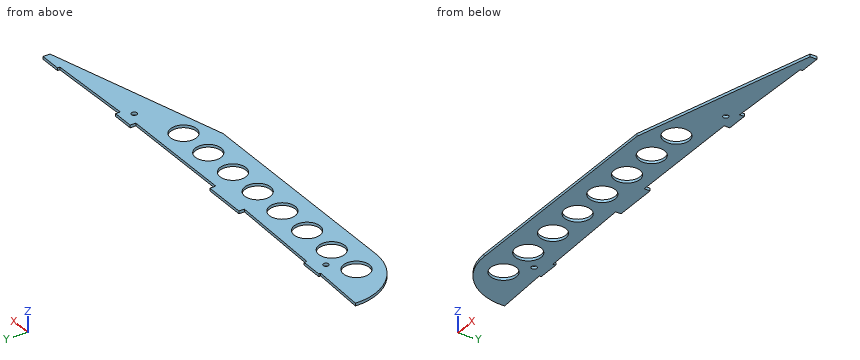
```python
from build123d import *

# Parameters (mm, degrees)
BOSS_EXTRUDE1_DEPTH      = 1.5875
BOSS_EXTRUDE1_DEPTH_BACK = 1.5875
CUT_EXTRUDE1_DEPTH       = 552.50665189
CUT_EXTRUDE1_DEPTH_BACK  = 552.50665189
SKETCH2_R                = 3.175
CUT_EXTRUDE2_DEPTH       = 2.54
CUT_EXTRUDE2_DEPTH_BACK  = 2.54
SKETCH3_R                = 15.24


with BuildPart() as part:
    # Sketch1 → Boss-Extrude1 (new, two sides: drawn at the far end of the back side and taken through both)
    with BuildSketch(Plane.XY.offset(-BOSS_EXTRUDE1_DEPTH_BACK)):
        with BuildLine():
            Line((331.479240226, -67.327812174), (547.379240226, -9.015530032))
            Line((547.379240226, -9.015530032), (547.379240226, -0.80358759))
            Line((547.379240226, -0.80358759), (521.979240226, -0.80358759))
            Line((521.979240226, -0.80358759), (521.979240226, -3.550327588))
            Line((521.979240226, -3.550327588), (420.379240226, -6.318039604))
            Line((420.379240226, -6.318039604), (420.379240226, -0.80358759))
            Line((420.379240226, -0.80358759), (394.979240226, -0.80358759))
            Line((394.979240226, -0.80358759), (394.979240226, -7.4329025))
            Line((394.979240226, -7.4329025), (255.21408059, -7.4329025))
            Line((255.21408059, -7.4329025), (255.21408059, -0.503629592))
            Line((255.21408059, -0.503629592), (204.41408059, -0.503629592))
            Line((204.41408059, -0.503629592), (204.41408059, -6.875812174))
            Line((204.41408059, -6.875812174), (90.223191735, -3.707270632))
            Line((90.223191735, -3.707270632), (90.223191735, -0.503629592))
            Line((90.223191735, -0.503629592), (64.823191735, -0.503629592))
            Line((64.823191735, -0.503629592), (64.823191735, -2.772070572))
            Line((64.823191735, -2.772070572), (0, 0))
            ThreePointArc((0, 0), (17.887759649, -47.42996384), (64.510168925, -67.327812174))
            Line((64.510168925, -67.327812174), (331.479240226, -67.327812174))
        make_face()
    extrude(amount=BOSS_EXTRUDE1_DEPTH + BOSS_EXTRUDE1_DEPTH_BACK)

    # Sketch2 → Cut-Extrude1 (cut, two sides: drawn at the far end of the back side and taken through both)
    with BuildSketch(Plane.XY.offset(-CUT_EXTRUDE1_DEPTH_BACK)):
        with Locations((410.219240226, -15.743629592)):
            Circle(SKETCH2_R)
        with Locations((74.939240226, -15.743629592)):
            Circle(SKETCH2_R)
    extrude(amount=CUT_EXTRUDE1_DEPTH + CUT_EXTRUDE1_DEPTH_BACK, mode=Mode.SUBTRACT)

    # Sketch3 → Cut-Extrude2 (cut, two sides: drawn at the far end of the back side and taken through both)
    with BuildSketch(Plane.XY.offset(-CUT_EXTRUDE2_DEPTH_BACK)):
        with BuildLine():
            ThreePointArc((79.242840924, -35.710884581), (94.482840924, -50.950884581), (109.722840924, -35.710884581))
            Line((109.722840924, -35.710884581), (79.242840924, -35.710884581))
        make_face()
        with BuildLine():
            Line((79.242840924, -35.710884581), (109.722840924, -35.710884581))
            ThreePointArc((109.722840924, -35.710884581), (94.482840924, -20.470884581), (79.242840924, -35.710884581))
        make_face()
        with BuildLine():
            ThreePointArc((368.802840924, -35.710884581), (353.562840924, -20.470884581), (338.322840924, -35.710884581))
            ThreePointArc((338.322840924, -35.710884581), (353.562840924, -50.950884581), (368.802840924, -35.710884581))
        make_face()
        with Locations((51.302840924, -35.710884581)):
            Circle(SKETCH3_R)
        with Locations((137.662840924, -35.710884581)):
            Circle(SKETCH3_R)
        with Locations((180.842840924, -35.710884581)):
            Circle(SKETCH3_R)
        with Locations((224.022840924, -35.710884581)):
            Circle(SKETCH3_R)
        with Locations((267.202840924, -35.710884581)):
            Circle(SKETCH3_R)
        with Locations((310.382840924, -35.710884581)):
            Circle(SKETCH3_R)
    extrude(amount=CUT_EXTRUDE2_DEPTH + CUT_EXTRUDE2_DEPTH_BACK, mode=Mode.SUBTRACT)


solid = part.part
```
Check sheet for the modelled part. Datum: model origin and axes. Units: mm. Coordinates: 2 decimals unless noted, no trailing zeros. Loops run counter-clockwise (first coordinate to the right, second up) from the corner with the lowest first, then second, coordinate; pieces in that order, holes last.
1) Sectioned sample at A-A (x = 311.5). Record the boundary of the cut face in (y, z).
2) Gauge pin test, flat ends, axial feed: pin 1 (1 mm diameter, centred on x = 342.5, z = 1, fed in from -Y); pin 2 (1.4 mm diameter, centred on y = -1.5, z = -0.5, fed in from -X); pin 3 (18.5 mm diameter, centred on x = 137.66, y = -35.71, fed in from -Z); pin 4 (10 mm diameter, centred on x = 410.22, y = -15.74, fed in from -Z). Record the tip position at first contact, or that the pin passes through.
3) Material ranges on probe 1 along Y at (x, z) = (182, -1.35); probe 2 along Y at (x, z) = (191, 0.55); probe 3 along Y at (x, z) = (71, 1.05), recorded low to high.
4) Sectioned sample at B-B (z = -1.1). Count the separate pieces of the cut face and the enclosed holes in it, and give its area (3 significant figures).
5) Sectioned sample at C-C (x = 56.5). Record the boundary of the cut face in (y, z), and give its area (3 significant figures).
Check sheet entries:
1. outline: (-67.33, -1.59) - (-50.91, -1.59) - (-50.91, 1.59) - (-67.33, 1.59) - close; (-20.51, -1.59) - (-7.43, -1.59) - (-7.43, 1.59) - (-20.51, 1.59) - close
2. pin 1: stops at y = -64.49
2. pin 2: stops at x = -0.06
2. pin 3: passes through
2. pin 4: stops at z = -1.59
3. probe 1: y = -67.33 to -50.91, -20.51 to -6.25
3. probe 2: y = -67.33 to -47.07, -24.35 to -6.5
3. probe 3: y = -67.33 to -0.5
4. separate pieces: 1
4. enclosed holes: 10
4. area: 21,500 mm2
5. outline: (-66.83, -1.59) - (-50.04, -1.59) - (-50.04, 1.59) - (-66.83, 1.59) - close; (-21.38, -1.59) - (-2.42, -1.59) - (-2.42, 1.59) - (-21.38, 1.59) - close
5. area: 114 mm2
